Build history of the part. All positions in model axes, mm. Face numbers are marked on the shaded views. A direction names the side the tool comes from. Give positions to 0.01 mm unless a question says otherwise; leave off trailing zeros. Loops run counter-clockwise (first coordinate to the right, second up) from the corner with the lowest first, then second, coordinate; pieces in that order, holes last. Notation, with made-up numbers: M 40,-23.75 L 79,-23.75 A15 ccw 79,-6.75 Z; hole C 2,-10.5 d5. An arc over 180 degrees is marked long. Put each result on its own line as item: value.
```python
from build123d import *

# Parameters (mm, degrees)
SKETCH1_R           = 2.2225
BOSS_EXTRUDE1_DEPTH = 0.79375
SKETCH2_R           = 1.5875
BOSS_EXTRUDE2_DEPTH = 7.62
CUT_EXTRUDE2_START  = -7.62
CUT_EXTRUDE2_DEPTH  = 7.62
FILLET1_R           = 0.635
FILLET2_R           = 0.381
CHAMFER1_SIZE       = 0.381


with BuildPart() as part:
    # Sketch1 → Boss-Extrude1 (new body)
    with BuildSketch(Plane(origin=(0, 0, 0), x_dir=(1, 0, 0), z_dir=(0, 1, 0))):
        with Locations(Location((0, 0, 0), (0, 0, 270))):
            Circle(SKETCH1_R)
    extrude(amount=BOSS_EXTRUDE1_DEPTH)

    # Sketch2 → Boss-Extrude2 (add)
    with BuildSketch(Plane.XZ):
        with Locations(Location((0, 0, 0), (0, 0, 90))):
            Circle(SKETCH2_R)
    extrude(amount=BOSS_EXTRUDE2_DEPTH)

    # Sketch3 → Cut-Extrude2 (cut)
    with BuildSketch(Plane.XZ.offset(7.62).offset(CUT_EXTRUDE2_START)):
        with BuildLine():
            Line((-0.586275376, 1.475275376), (-0.586275376, 0.586275376))
            Line((-0.586275376, 0.586275376), (-1.475275376, 0.586275376))
            ThreePointArc((-1.475275376, 0.586275376), (-1.122532015, 1.122532015), (-0.586275376, 1.475275376))
        make_face()
        with BuildLine():
            Line((-1.475275376, -0.586275376), (-0.586275376, -0.586275376))
            Line((-0.586275376, -0.586275376), (-0.586275376, -1.475275376))
            ThreePointArc((-0.586275376, -1.475275376), (-1.122532015, -1.122532015), (-1.475275376, -0.586275376))
        make_face()
        with BuildLine():
            Line((0.586275376, 1.475275376), (0.586275376, 0.586275376))
            Line((0.586275376, 0.586275376), (1.475275376, 0.586275376))
            ThreePointArc((1.475275376, 0.586275376), (1.122532015, 1.122532015), (0.586275376, 1.475275376))
        make_face()
        with BuildLine():
            Line((0.586275376, -1.475275376), (0.586275376, -0.586275376))
            Line((0.586275376, -0.586275376), (1.475275376, -0.586275376))
            ThreePointArc((1.475275376, -0.586275376), (1.122532015, -1.122532015), (0.586275376, -1.475275376))
        make_face()
    extrude(amount=CUT_EXTRUDE2_DEPTH, mode=Mode.SUBTRACT)

    # Fillet1
    fillet1_edges = [part.edges().sort_by_distance(p)[0] for p in [
        (-0.586275376, -3.81, -0.586275376),
        (0.586275376, -3.81, 0.586275376),
        (0.586275376, -3.81, -0.586275376),
        (-0.586275376, -3.81, 0.586275376),
    ]]
    fillet(fillet1_edges, radius=FILLET1_R)

    # Fillet2
    fillet2_edges = [part.edges().sort_by_distance(p)[0] for p in [
        (-1.5875, -7.62, 0),
        (0, -7.62, -1.5875),
        (1.5875, -7.62, 0),
        (0, -7.62, 1.5875),
    ]]
    fillet(fillet2_edges, radius=FILLET2_R)

    # Chamfer1
    chamfer1_edges = [part.edges().sort_by_distance(p)[0] for p in [
        (0, 0, -2.2225),
    ]]
    chamfer(chamfer1_edges, length=CHAMFER1_SIZE)


solid = part.part
```
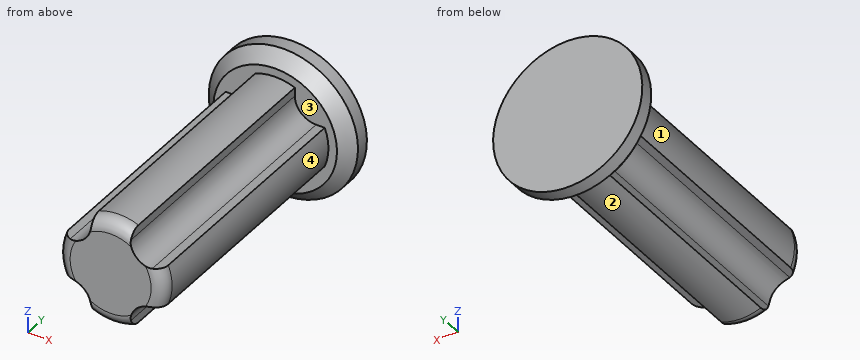
Q1. Tool access for the marked faces 1, 2, 3 and 4: list every direction of +Z, -Z, +X, -X, +Y, -Y with a clear straight run to the whole face (end or side of a thin tool).
Here are the results:
face 1: -X, -Y
face 2: -Z, -Y
face 3: -Y
face 4: +X, -Y
Q2. Slice it at B-B (z = 0). List the corners of the cut face in (x, y).
Here are the results:
outline: M -2.22,0.38 L -1.84,0 L -1.59,0 L -1.59,-7.24 A0.38 ccw -1.21,-7.62 L 1.21,-7.62 A0.38 ccw 1.59,-7.24 L 1.59,0 L 1.84,0 L 2.22,0.38 L 2.22,0.79 L -2.22,0.79 Z
Q3. Slice it at A-A (x = 0). List the corners of the cut face in (y, z).
Here are the results:
outline: M -7.62,-1.21 A0.38 ccw -7.24,-1.59 L 0,-1.59 L 0,-1.84 L 0.38,-2.22 L 0.79,-2.22 L 0.79,2.22 L 0.38,2.22 L 0,1.84 L 0,1.59 L -7.24,1.59 A0.38 ccw -7.62,1.21 Z
Q4. Drop flat-ended pins along their axis: pin 1 Ø1.5 at (y, z) = (-2, -0.5) entering from -X; pin 2 Ø1.5 at (x, y) = (0, -3.5) entering from +Z. Give the stop position or say it passes through.
Here are the results:
pin 1: x = -1.59
pin 2: z = 1.59
Q5. Probe line 1 (Z direction, x = 1.2, y = -2.5); line 2 (Y direction, x = -0.85, z = -0.8). List the from-to ranges inside material, lowest first. Write a range as from..to.
Here are the results:
line 1: -0.59..0.59
line 2: 0..0.79
